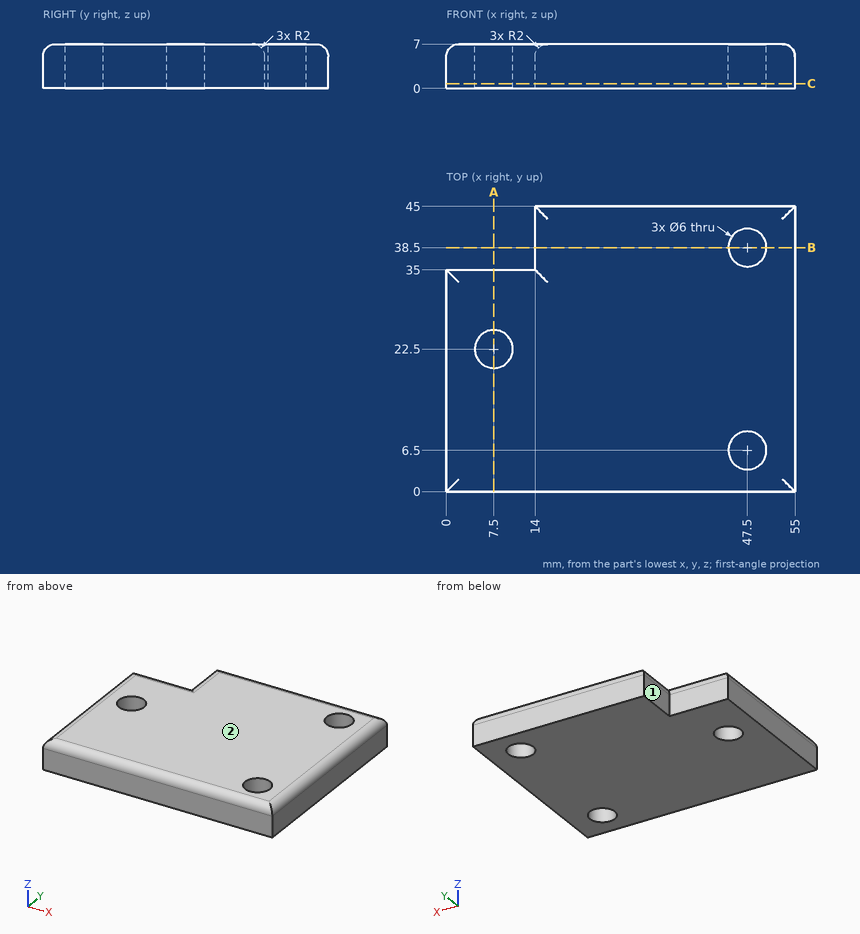
Verification items for this drawing (mm, ordinates from the low corner). A direction names the side the tool comes from. Coordinates: 2 decimals unless noted, no trailing zeros. Loops run counter-clockwise (first coordinate to the right, second up) from the corner with the lowest first, then second, coordinate; pieces in that order, holes last. Notation, with made-up numbers: (-7, -30.5) - (32, -30.5) arc R16 ccw to (32, -19.5) - close; hole circle Ø8 at (0.25, 29). An arc over 180 degrees is marked (long way). Use one line per item in the form item = value. Start each with the question number.
Item 1: Section check A-A, the plane x = 7.5. Enter the section's corners in (y, z).
Item 2: Thickness scan on probe 1 along X at (y, z) = (22.5, 3); probe 2 along Y at (x, z) = (45.5, 5); probe 3 along Y at (x, z) = (49, 2). Record the ranges inside material, lowest first.
Item 3: Section check C-C, the plane z = 0.75. Enter the section's corners in (x, y).
Item 4: Section check B-B, the plane y = 38.5. Enter the section's corners in (x, z), and give its area (3 significant figures).
Item 5: Tool access check on the marked faces 1 and 2. Record the directions out of +Z, -Z, +X, -X, +Y, -Y that give a thin tool (end or side, any length) a straight path to the whole face; none if there is none.
Item 6: Gauge pin test, flat ends, axial feed: pin 1 (8 mm diameter, centred on x = 47, y = 32, fed in from -Z); pin 2 (5.5 mm diameter, centred on x = 47.5, y = 6.5, fed in from -Z); pin 3 (2.5 mm diameter, centred on y = 40, z = 2, fed in from -X); pin 4 (1.5 mm diameter, centred on x = 7.5, z = 3.5, fed in from +Y). Record the tip position at first contact, or that the pin passes through.
Computed:
q1.outline = (0, 0) - (19.5, 0) - (19.5, 7) - (2, 7) arc R2 ccw to (0, 5) - close; (25.5, 0) - (35, 0) - (35, 5) arc R2 ccw to (33, 7) - (25.5, 7) - close
q2.probe_1 = 0 to 4.5, 10.5 to 55
q2.probe_2 = 0 to 4.26, 8.74 to 36.26, 40.74 to 45
q2.probe_3 = 0 to 3.9, 9.1 to 35.9, 41.1 to 45
q3.outline = (0, 0) - (55, 0) - (55, 45) - (14, 45) - (14, 35) - (0, 35) - close; hole circle Ø6 at (7.5, 22.5); hole circle Ø6 at (47.5, 6.5); hole circle Ø6 at (47.5, 38.5)
q4.outline = (14, 0) - (44.5, 0) - (44.5, 7) - (16, 7) arc R2 ccw to (14, 5) - close; (50.5, 0) - (55, 0) - (55, 5) arc R2 ccw to (53, 7) - (50.5, 7) - close
q4.area = 243 mm2
q5.face_1 = +Z, -Z, -X, +Y
q5.face_2 = +Z, +X, -X, +Y, -Y
q6.pin_1 = 0
q6.pin_2 = through
q6.pin_3 = 14
q6.pin_4 = 35
